Part model, mm, in its own coordinate system. A direction names the side the tool comes from. Give positions to 0.01 mm unless a question says otherwise; leave off trailing zeros. Order: outer loops, then holes, each group sorted by start corner. A loop starts at its lowest first (then second) coordinate and runs counter-clockwise, first axis right, second up. Notation, with made-up numbers: (-20.5, 87.25) - (-6.5, 87.25) arc R21 ccw to (-6.5, 120.25) - close; hole circle Ø10 at (-16, -34). An arc over 180 degrees is marked (long way). One line per item, written item: value.
```python
from build123d import *

# Parameters (mm, degrees)
F0_W     = 40
F0_H     = 40
F0_R     = 12.5
F3_ANGLE = 90


with BuildPart() as f2:
    # F2: sweep along a path in F1
    with BuildLine(Plane.XZ) as f2_path:
        Line((0, 0), (0, 5))
        ThreePointArc((0, 5), (7.3223304703, 22.6776695297), (25, 30))
        Line((25, 30), (50, 30))
    # F0 (on Top) → F2 (sweep)
    with BuildSketch(Plane.XY):
        Rectangle(F0_W, F0_H)
        Circle(F0_R, mode=Mode.SUBTRACT)
    sweep(path=f2_path.line)


with BuildPart() as f2_1:
    # F3: moved
    add(f2.part.rotate(Axis((0, -20, 0), (1, 0, 0)), F3_ANGLE))


solid = f2_1.part
```
1) Mould opens along X. For faces 1 (the cylindrical face through (5.77, -22.53, 8.91)), 2 (the flat face through (38, -30, 20)), 3 (the cylindrical face through (21, -28, 20)) say: released by +X, released by -X, zero draft, split by the parting line, or undercut.
Outcome:
face 1: undercut
face 2: zero draft
face 3: released by +X
2) Cut at A-A, the plane z = 20. Give the cut face in (x, y), then the cut area to 3 significant figures.
Outcome:
outline: (-20, -25) arc R45 ccw to (25, -70) - (50, -70) - (50, -62.5) - (25, -62.5) arc R37.5 cw to (-12.5, -25) - (-12.5, -20) - (-20, -20) - close; (12.5, -25) arc R12.5 ccw to (25, -37.5) - (50, -37.5) - (50, -30) - (25, -30) arc R5 cw to (20, -25) - (20, -20) - (12.5, -20) - close
area: 1,040 mm^2
3) Cut at D-D, the plane z = 30. Give the cut face in (x, y), then the cut area to 3 significant figures.
Outcome:
outline: (-20, -25) arc R45 ccw to (25, -70) - (50, -70) - (50, -57.5) - (25, -57.5) arc R32.5 cw to (-7.5, -25) - (-7.5, -20) - (-20, -20) - close; (7.5, -25) arc R17.5 ccw to (25, -42.5) - (50, -42.5) - (50, -30) - (25, -30) arc R5 cw to (20, -25) - (20, -20) - (7.5, -20) - close
area: 1,730 mm^2
4) Cut at C-C, the plane z = 5.5. Give the cut face in (x, y), then the cut area to 3 significant figures.
Outcome:
outline: (-20, -25) arc R45 ccw to (25, -70) - (50, -70) - (50, -30) - (25, -30) arc R5 cw to (20, -25) - (20, -20) - (-20, -20) - close
area: 2,770 mm^2
5) Drill centre lines: line 1 along Z through (x, y) = (0, -23.8); line 2 along Z through (x, y) = (22.5, -40); line 3 along X through (y, z) = (-22, 18). Where is each one in solid material? Low to high. Write a range as from..to.
Outcome:
line 1: z = 0..7.5, 32.5..40
line 2: z = 0..12.23, 27.77..40
line 3: x = -20..-12.34, 12.34..20
6) Pin check, flat tips, straight feed: pin 1 (20 mm diameter, centred on x = 32, z = 12.5, fed in from +Y); pin 2 (3 mm diameter, centred on x = -6.5, z = 28.5, fed in from -Y); pin 3 (2 mm diameter, centred on x = 36, z = 5.5, fed in from +Y). Stop position of each tip, or through.
Outcome:
pin 1: stops at y = -29
pin 2: stops at y = -58.54
pin 3: stops at y = -30
7) Which spindle directions (+Z, -Z, +X, -X, +Y, -Y) get a long thin tool onto all of the face, cutting with end or side? Do faces 4 (the flat face through (-9, -20, 29)), 5 (the cylindrical face through (37.675, -59.92, 12.394)), 6 (the flat face through (20, -23, 20)). Say none if no direction does.
Outcome:
face 4: +Z, -Z, +X, -X, +Y
face 5: +X
face 6: +Z, -Z, +X, +Y
8) Cut at B-B, the plane x = 38. Give the cut face in (y, z).
Outcome:
outline: (-70, 0) - (-30, 0) - (-30, 40) - (-70, 40) - close; hole circle Ø25 at (-50, 20)
